Autodesk Inventor part; units mm, degrees
ref_plane "YZ Plane" through (0, 0, 0) normal (1, 0, 0) x (0, 1, 0)
ref_plane "XZ Plane" through (0, 0, 0) normal (0, 1, 0) x (-1, 0, 0)
ref_plane "XY Plane" through (0, 0, 0) normal (0, 0, 1) x (1, 0, 0)
sketch "Skizze1" plane through (0, 0, 0) normal (0, 0, 1) x (1, 0, 0)
  line L0 (-25, 25) -> (25, 25)
  line L1 (25, 25) -> (25, -25)
  line L2 (25, -25) -> (-25, -25)
  line L3 (-25, -25) -> (-25, 25)
  line L4 (-25, 25) -> (25, -25) construction
  line L5 (25, 25) -> (-25, -25) construction
  point P0 (0, 0)
  dimension "d0" = 50
  dimension "d1" = 50
extrude "Extrusion1" add sketch "Skizze1" along normal blind 2
chamfer "Fase1" distance 2 distance2 3 1 edges at (0, 25, 0) measured on face at (8.3333, 25, 0.6667)
properties part number "plate90"
Design review of the part built by this model. Coordinates are the model's own, in mm. Round coordinates to 2 decimals unless told otherwise and drop trailing zeros. Write each loop counter-clockwise with the first axis right and the second up, starting at its lowest first coordinate (ties: lowest second). Pieces come first, ordered by that corner, then holes.
Item 1: Wall thickness on L1, parallel to Y at x = 18.5, z = 1.75; L2, parallel to Y at x = 16, z = 1.2: over which ranges is each line inside the solid? List them lowest first.
Item 2: For pin 1 Ø10 at (x, y) = (0, 12) entering from -Z, flat-tipped, find the tip position at first contact; note if it passes through.
Item 3: Consider section B-B on z = 0.6. Give the boundary of the cut face in (x, y), and give its area (3 significant figures).
Check values:
1. L1: y = -25 to 24.63
1. L2: y = -25 to 23.8
2. pin 1: stops at z = 0
3. outline: (-25, -25) - (25, -25) - (25, 22.9) - (-25, 22.9) - close
3. area: 2,400 mm2
